Verification items for the finished model (mm, model axes). Round coordinates to 2 decimals unless told otherwise and drop trailing zeros. Order: outer loops, then holes, each group sorted by start corner. A loop starts at its lowest first (then second) coordinate and runs counter-clockwise, first axis right, second up. Notation, with made-up numbers: (77.5, 56) -> (101.5, 56) arc R19 cw to (101.5, 61) -> close; hole circle Ø6 at (-2, 2.25). An arc over 180 degrees is marked (long way). Return JSON: item names as keys, results as strings. Group by question number.
Item 1: Sectioned sample at A-A on z = -35. Give the number of separate pieces and of enclosed holes in the cut face, plus the area to 3 significant figures.
Item 2: Sectioned sample at B-B on z = -64.5. Record the cut outline in (x, y), plus the area to 3 significant figures.
Item 3: Sectioned sample at C-C on x = 92.5. Record the cut outline in (y, z).
Item 4: Scan lines: probe 1 along Z at (x, y) = (27, 1.7); probe 2 along Z at (x, y) = (127, 2.3); probe 3 along X at (y, z) = (1, -8). Record each from-to range of solid material in increasing order. Write a range as from..to.
Item 5: Depth check by flat-ended pin: pin 1 Ø2 at (y, z) = (2, -116.5) entering from -X; pin 2 Ø2.5 at (x, y) = (108.5, 3.5) entering from -Z; pin 3 Ø1 at (y, z) = (1.5, -77.5) entering from +X. Enter the tip coordinate at first touch or a pass-through.
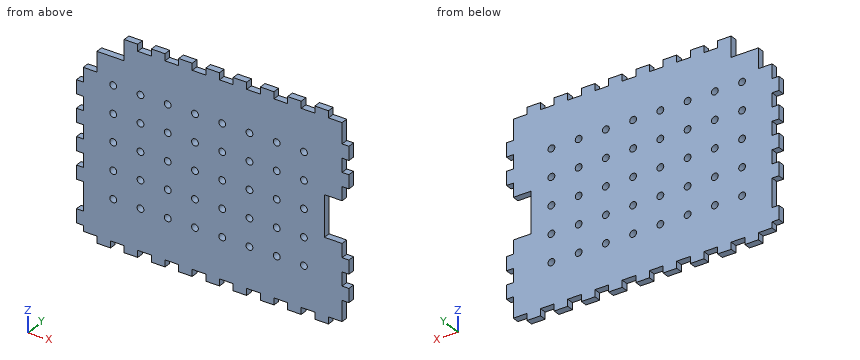
```python
from build123d import *

# Parameters (mm, degrees)
SALIENTE_EXTRUIR1_DEPTH = 5
CROQUIS2_R              = 2.5
CORTAR_EXTRUIR1_DEPTH   = 10


with BuildPart() as part:
    # Croquis1 → Saliente-Extruir1 (new body)
    with BuildSketch(Plane(origin=(0, 0, 0), x_dir=(1, 0, 0), z_dir=(0, 1, 0))):
        Polygon((15, 5), (15, 0), (25, 0), (25, 5), (35, 5), (35, 0), (45, 0), (45, 5), (55, 5), (55, 0), (65, 0), (65, 5), (75, 5), (75, 0), (85, 0), (85, 5), (95, 5), (95, 0), (105, 0), (105, 5), (115, 5), (115, 0), (125, 0), (125, 5), (135, 5), (135, 0), (145, 0), (145, 5), (155, 5), (155, 0), (165, 0), (165, 5), (175, 5), (175, 0), (185, 0), (185, 5), (195, 5), (195, 20), (200, 20), (200, 30), (195, 30), (195, 40), (200, 40), (200, 50), (195, 50), (195, 60), (200, 60), (200, 70), (195, 70), (195, 80), (200, 80), (200, 90), (195, 90), (195, 100), (200, 100), (200, 110), (195, 110), (195, 120), (200, 120), (200, 130), (195, 130), (195, 145), (185, 145), (185, 150), (175, 150), (175, 145), (165, 145), (165, 150), (155, 150), (155, 145), (145, 145), (145, 150), (135, 150), (135, 145), (125, 145), (125, 150), (115, 150), (115, 145), (105, 145), (105, 150), (95, 150), (95, 145), (85, 145), (85, 150), (75, 150), (75, 145), (65, 145), (65, 150), (55, 150), (55, 145), (45, 145), (45, 150), (35, 150), (35, 145), (25, 145), (25, 150), (15, 150), (15, 145), (5, 145), (5, 140.75), (0, 140.75), (0, 130.75), (5, 130.75), (5, 110), (0, 110), (0, 100), (5, 100), (5, 90), (0, 90), (0, 80), (5, 80), (5, 70), (0, 70), (0, 60), (5, 60), (5, 50), (0, 50), (0, 40), (5, 40), (5, 19.25), (0, 19.25), (0, 9.25), (5, 9.25), (5, 5), align=None)
    extrude(amount=SALIENTE_EXTRUIR1_DEPTH)

    # Croquis2 → Cortar-Extruir1 (cut)
    with BuildSketch(Plane(origin=(0, 5, 0), x_dir=(1, 0, 0), z_dir=(0, 1, 0))):
        with Locations((27, 115)):
            Circle(CROQUIS2_R)
        with Locations((47, 115)):
            Circle(CROQUIS2_R)
        with Locations((67, 115)):
            Circle(CROQUIS2_R)
        with Locations((87, 115)):
            Circle(CROQUIS2_R)
        with Locations((107, 115)):
            Circle(CROQUIS2_R)
        with Locations((127, 115)):
            Circle(CROQUIS2_R)
        with Locations((147, 115)):
            Circle(CROQUIS2_R)
        with Locations((167, 115)):
            Circle(CROQUIS2_R)
        with Locations((47, 95)):
            Circle(CROQUIS2_R)
        with Locations((67, 95)):
            Circle(CROQUIS2_R)
        with Locations((87, 95)):
            Circle(CROQUIS2_R)
        with Locations((107, 95)):
            Circle(CROQUIS2_R)
        with Locations((127, 95)):
            Circle(CROQUIS2_R)
        with Locations((147, 95)):
            Circle(CROQUIS2_R)
        with Locations((167, 95)):
            Circle(CROQUIS2_R)
        with Locations((47, 75)):
            Circle(CROQUIS2_R)
        with Locations((67, 75)):
            Circle(CROQUIS2_R)
        with Locations((87, 75)):
            Circle(CROQUIS2_R)
        with Locations((107, 75)):
            Circle(CROQUIS2_R)
        with Locations((127, 75)):
            Circle(CROQUIS2_R)
        with Locations((147, 75)):
            Circle(CROQUIS2_R)
        with Locations((167, 75)):
            Circle(CROQUIS2_R)
        with Locations((47, 55)):
            Circle(CROQUIS2_R)
        with Locations((67, 55)):
            Circle(CROQUIS2_R)
        with Locations((87, 55)):
            Circle(CROQUIS2_R)
        with Locations((107, 55)):
            Circle(CROQUIS2_R)
        with Locations((127, 55)):
            Circle(CROQUIS2_R)
        with Locations((147, 55)):
            Circle(CROQUIS2_R)
        with Locations((167, 55)):
            Circle(CROQUIS2_R)
        with Locations((47, 35)):
            Circle(CROQUIS2_R)
        with Locations((67, 35)):
            Circle(CROQUIS2_R)
        with Locations((87, 35)):
            Circle(CROQUIS2_R)
        with Locations((107, 35)):
            Circle(CROQUIS2_R)
        with Locations((127, 35)):
            Circle(CROQUIS2_R)
        with Locations((147, 35)):
            Circle(CROQUIS2_R)
        with Locations((167, 35)):
            Circle(CROQUIS2_R)
        with Locations((27, 95)):
            Circle(CROQUIS2_R)
        with Locations((27, 75)):
            Circle(CROQUIS2_R)
        with Locations((27, 55)):
            Circle(CROQUIS2_R)
        with Locations((27, 35)):
            Circle(CROQUIS2_R)
        Polygon((5, 29.625), (5, 19.25), (0, 19.25), (0, 9.25), (5, 9.25), (5, 5), (15, 5), (15, 0), (25, 0), (25, 5), (35, 5), (35, 15), (15, 15), (15, 29.625), align=None)
        Polygon((195, 90), (200, 90), (200, 80), (195, 80), (195, 70), (200, 70), (200, 60), (195, 60), (182, 60), (182, 90), align=None)
    extrude(amount=-CORTAR_EXTRUIR1_DEPTH, mode=Mode.SUBTRACT)


solid = part.part
```
Recorded:
{
 "1": {"separate pieces": "9", "enclosed holes": "0", "area": "750 mm²"},
 "2": {"outline": "(0, 0) -> (182, 0) -> (182, 5) -> (0, 5) -> close", "area": "910 mm²"},
 "3": {"outline": "(0, -145) -> (5, -145) -> (5, -5) -> (0, -5) -> close"},
 "4": {"probe 1": "-145..-117.5, -112.5..-97.5, -92.5..-77.5, -72.5..-57.5, -52.5..-37.5, -32.5..-15", "probe 2": "-145..-117.5, -112.5..-97.5, -92.5..-77.5, -72.5..-57.5, -52.5..-37.5, -32.5..-5", "probe 3": "35..195"},
 "5": {"pin 1": "x = 5", "pin 2": "z = -145", "pin 3": "x = 182"}
}
